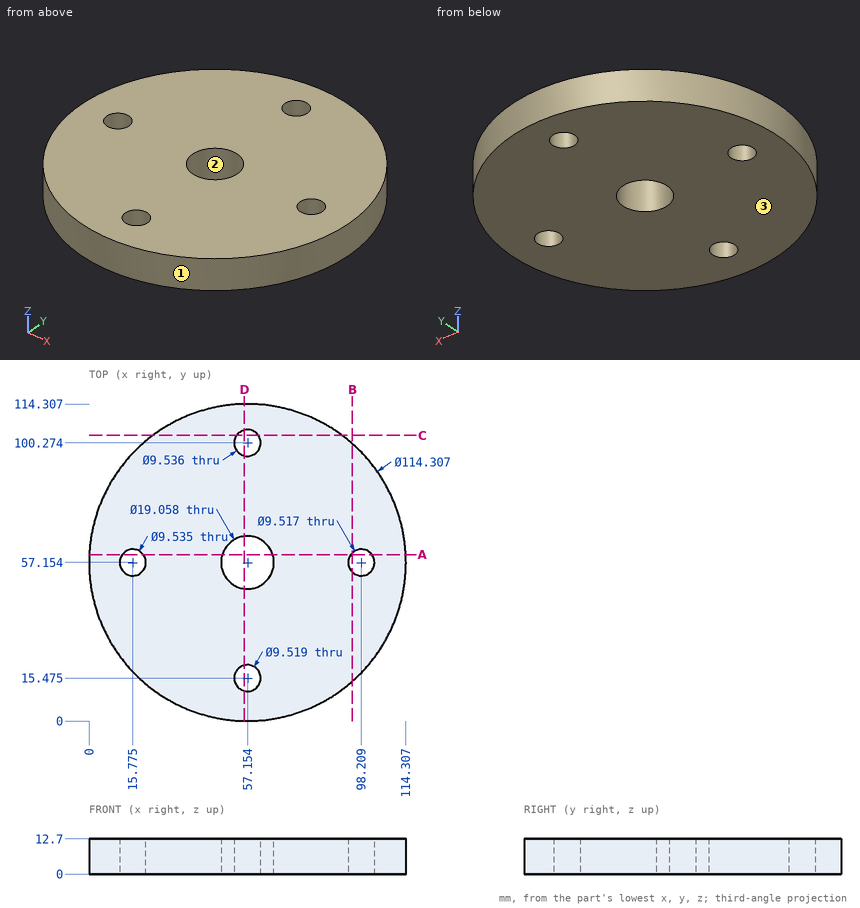
Part print with two shaded views. Sizes in mm from the minimum x, y, z corner. Round coordinates to 2 decimals unless told otherwise and drop trailing zeros. Write each loop counter-clockwise with the first axis right and the second up, starting at its lowest first coordinate (ties: lowest second). Pieces come first, ordered by that corner, then holes. Notation, with made-up numbers: (81.25, 83) -> (138.25, 83) arc R20 ccw to (138.25, 113) -> close; hole circle Ø1 at (-14, 34.25). An arc over 180 degrees is marked (long way). Put each result on its own line as item: value.
Item 1: Slice it at A-A, the plane y = 60. Give the cut face in (x, z).
Here are the results:
outline: (0.07, 0) -> (11.95, 0) -> (11.95, 12.7) -> (0.07, 12.7) -> close; (19.6, 0) -> (48.06, 0) -> (48.06, 12.7) -> (19.6, 12.7) -> close; (66.25, 0) -> (94.4, 0) -> (94.4, 12.7) -> (66.25, 12.7) -> close; (102.02, 0) -> (114.24, 0) -> (114.24, 12.7) -> (102.02, 12.7) -> close
Item 2: Slice it at D-D, the plane x = 56. Give the cut face in (y, z) (1 decimal).
Here are the results:
outline: (0, 0) -> (10.9, 0) -> (10.9, 12.7) -> (0, 12.7) -> close; (20.1, 0) -> (47.7, 0) -> (47.7, 12.7) -> (20.1, 12.7) -> close; (66.6, 0) -> (95.6, 0) -> (95.6, 12.7) -> (66.6, 12.7) -> close; (104.9, 0) -> (114.3, 0) -> (114.3, 12.7) -> (104.9, 12.7) -> close
Item 3: Wall check: probe 1 along X at (y, z) = (57, 11) (1 decimal); probe 2 along Y at (x, z) = (99, 10.5) (1 decimal); probe 3 along Y at (x, z) = (51, 9.75) (1 decimal). Give the ranges that are in metal, low to high. Write a range as from..to.
Here are the results:
probe 1: x = 0..11, 20.5..47.6, 66.7..93.5, 103..114.3
probe 2: y = 18.2..52.5, 61.8..96.1
probe 3: y = 0.3..49.9, 64.4..114
Item 4: Two-plate mould, pull along X, no slides. Class the marked faces 1, 2 and 3: pulls with the +X half, pulls with the -X half, needs draft (parallel to the pull), parting line crosses it, or undercut.
Here are the results:
face 1: parting line crosses it
face 2: undercut
face 3: needs draft
Item 5: Flat gauge pins, fed straight in: P1, Ø1, axis at x = 48, z = 5.5, coming from the -Y side; P2, Ø5, axis at x = 82, z = 10.5, coming from the -Y side; P3, Ø4, axis at x = 100.5, z = 10, coming from the -Y side (1 decimal). Where does each tip first touch, or does it go through?
Here are the results:
P1: stops at y = 0.66
P2: stops at y = 4.55
P3: stops at y = 17.7
Item 6: Slice it at B-B, the plane x = 95. Give the cut face in (y, z).
Here are the results:
outline: (14.33, 0) -> (53.64, 0) -> (53.64, 12.7) -> (14.33, 12.7) -> close; (60.67, 0) -> (99.98, 0) -> (99.98, 12.7) -> (60.67, 12.7) -> close
Item 7: Slice it at C-C, the plane y = 103. Give the cut face in (x, z) (1 decimal).
Here are the results:
outline: (23, 0) -> (53.2, 0) -> (53.2, 12.7) -> (23, 12.7) -> close; (61.1, 0) -> (91.3, 0) -> (91.3, 12.7) -> (61.1, 12.7) -> close
